Can you work these out from the model? Positions are in its coordinate system, mm. A direction names the side the tool comes from. Give positions to 0.01 mm unless a question says otherwise; leave off trailing zeros. Write each loop counter-clockwise with the first axis right and the second up, starting at its lowest first coordinate (ties: lowest second). Pieces come first, ordered by that corner, then holes.
1. If I drill on probe 1 along Y at (x, z) = (0, 1) (3 decimals); probe 2 along Y at (x, z) = (1.75, 0.4); probe 3 along Z at (x, y) = (4.5, 1), over which ranges is the centre line in solid material (lowest first)?
2. Suppose I cut it at B-B (z = 0.3). Please give me the cut outline in (x, y).
3. On a 3-axis mill with a long thin cutter (end or side, diameter ignored), from which of +Z, -Z, +X, -X, +Y, -Y can I reach the whole of each face in a straight line? I mean faces 1 (the flat face through (2, -2, 2)), 2 (the cylindrical face through (-2.893, -2.653, 1.24)). Say none if no direction works.
4. Thinking about a two-plate mould opening in Y: for faces 3 (the flat face through (2.24, 0.06, 0)), 4 (the flat face through (-3.88, -2.28, 0.25)), 5 (the flat face through (-3.915, 2.218, 0.246)), 6 (the cylindrical face through (1.26, 1.64, 0.99)), which applies, pulls with the +Y half, pulls with the -Y half, needs draft (parallel to the pull), parting line crosses it, or undercut?
5. Suppose I cut it at A-A (x = 0). Please give me the cut outline in (y, z) (3 decimals).
6. I'm going to push flat-ended pins straight in: pin 1 (1.5 mm diameter, centred on x = 4, y = -2, fed in from +Z); pin 2 (1 mm diameter, centred on x = 1, y = 1, fed in from -Z). Where does each tip first touch, or does it pass through?
7. Suppose I cut it at D-D (x = 2.25). Please give me the cut outline in (y, z), and give its area (3 significant figures).
8. Suppose I cut it at C-C (y = 0.75). Please give me the cut outline in (x, z), and give its area (3 significant figures).
Autodesk Inventor part; units mm, degrees
ref_plane "YZ Plane" through (0, 0, 0) normal (1, 0, 0) x (0, 1, 0)
ref_plane "XZ Plane" through (0, 0, 0) normal (0, 1, 0) x (-1, 0, 0)
ref_plane "XY Plane" through (0, 0, 0) normal (0, 0, 1) x (1, 0, 0)
sketch "スケッチ1" plane through (0, 0, 0) normal (0, 0, 1) x (1, 0, 0)
  line L0 (5.1962, 0) -> (2.5981, -4.5)
  line L1 (2.5981, -4.5) -> (-2.5981, -4.5)
  line L2 (-2.5981, -4.5) -> (-5.1962, 0)
  line L3 (-5.1962, 0) -> (-2.5981, 4.5)
  line L4 (-2.5981, 4.5) -> (2.5981, 4.5)
  line L5 (2.5981, 4.5) -> (5.1962, 0)
  point P0 (0, 0)
  point P1 (0, 0)
  dimension "d0" = 9
extrude "押し出し1" add sketch "スケッチ1" along normal blind 0.5
sketch "スケッチ2" plane through (0, 0, 0.5) normal (0, 0, 1) x (1, 0, 0)
  circle A0 centre (0, 0) radius 3.925
  dimension "d3" = 7.85
extrude "押し出し2" add sketch "スケッチ2" along normal blind 1.5
sketch "スケッチ3" plane through (0, 0, 2) normal (0, 0, 1) x (1, 0, 0)
  point P0 (0, 0)
hole "穴1" at (0, 0, 2) direction (0, 0, -1) diameter 4.134 depth 2
properties part number "TF-M5-2"
Checks:
1. probe 1: y = -3.925 to -2.067, 2.067 to 3.925
1. probe 2: y = -4.5 to -1.1, 1.1 to 4.5
1. probe 3: z = 0 to 0.5
2. outline: (-5.2, 0) - (-2.6, -4.5) - (2.6, -4.5) - (5.2, 0) - (2.6, 4.5) - (-2.6, 4.5) - close; hole circle Ø4.13 at (0, 0)
3. face 1: +Z, +X, -X, +Y, -Y
3. face 2: +Z
4. face 3: needs draft
4. face 4: pulls with the -Y half
4. face 5: pulls with the +Y half
4. face 6: undercut
5. outline: (-4.5, 0) - (-2.067, 0) - (-2.067, 2) - (-3.925, 2) - (-3.925, 0.5) - (-4.5, 0.5) - close; (2.067, 0) - (4.5, 0) - (4.5, 0.5) - (3.925, 0.5) - (3.925, 2) - (2.067, 2) - close
6. pin 1: stops at z = 2
6. pin 2: passes through
7. outline: (-4.5, 0) - (4.5, 0) - (4.5, 0.5) - (3.22, 0.5) - (3.22, 2) - (-3.22, 2) - (-3.22, 0.5) - (-4.5, 0.5) - close
7. area: 14.1 mm2
8. outline: (-4.76, 0) - (-1.93, 0) - (-1.93, 2) - (-3.85, 2) - (-3.85, 0.5) - (-4.76, 0.5) - close; (1.93, 0) - (4.76, 0) - (4.76, 0.5) - (3.85, 0.5) - (3.85, 2) - (1.93, 2) - close
8. area: 8.62 mm2
